from build123d import *

# Parameters (mm, degrees)
CROQUIS1_R              = 5.5
SALIENTE_EXTRUIR1_DEPTH = 4


with BuildPart() as part:
    # Croquis1 → Saliente-Extruir1 (new body)
    with BuildSketch(Plane.XY):
        Polygon((2.080750103, 8.567708442), (-6.379478111, 6.085836669), (-8.460228214, -2.481871773), (-2.080750103, -8.567708442), (6.379478111, -6.085836669), (8.460228214, 2.481871773), align=None)
        Circle(CROQUIS1_R, mode=Mode.SUBTRACT)
    extrude(amount=-SALIENTE_EXTRUIR1_DEPTH)


solid = part.part
Geometry check sheet. Reference: the model listing, model coordinates, mm. Round coordinates to 2 decimals unless told otherwise and drop trailing zeros. Order: outer loops, then holes, each group sorted by start corner. A loop starts at its lowest first (then second) coordinate and runs counter-clockwise, first axis right, second up. Notation, with made-up numbers: (62, -25.75) - (66, -25.75) arc R37 ccw to (66, 13.25) - close; hole circle Ø6 at (27, 65). An arc over 180 degrees is marked (long way). One line per question, with ' | ' between items. Start each with the question number.
(1) Depth check by flat-ended pin: pin 1 Ø1 at (x, z) = (-3.5, -3.5) entering from +Y; pin 2 Ø2 at (y, z) = (0, -0.5) entering from -X. Enter the tip coordinate at first touch or a pass-through.
(2) Sectioned sample at C-C on x = 0. Record the cut outline in (y, z).
(3) Sectioned sample at D-D on x = 6. Record the cut outline in (y, z), and give its area (3 significant figures).
(4) Sectioned sample at B-B on z = -0.85. Record the cut outline in (x, y).
(5) Sectioned sample at A-A on y = -1.25. Record the cut outline in (x, z).
(6) Thickness scan on L1, parallel to Y at x = 0, z = -1.15; L2, parallel to X at y = -4.5, z = -0.65; L3, parallel to Y at x = -2.75, z = -1.6. Record the ranges inside material, lowest first. Write a range as [from, to].
(7) Release check for a two-part mould opening along Y. For faces 1 (the cylindrical face through (-1.19, -5.37, -1.97)), 2 (the flat face through (5.32, 5.48, -1.97)), 3 (the flat face through (7.405, -1.862, -1.972)) record: released by +Y, released by -Y, zero draft, split by the parting line, or undercut.
Conclusion:
1) pin 1: stops at y = 7.08 | pin 2: stops at x = -8.1
2) outline: (-7.96, -4) - (-5.5, -4) - (-5.5, 0) - (-7.96, 0) - close; (5.5, -4) - (7.96, -4) - (7.96, 0) - (5.5, 0) - close
3) outline: (-6.2, -4) - (4.83, -4) - (4.83, 0) - (-6.2, 0) - close | area: 44.1 mm2
4) outline: (-8.46, -2.48) - (-2.08, -8.57) - (6.38, -6.09) - (8.46, 2.48) - (2.08, 8.57) - (-6.38, 6.09) - close; hole circle Ø11 at (0, 0)
5) outline: (-8.16, -4) - (-5.36, -4) - (-5.36, 0) - (-8.16, 0) - close; (5.36, -4) - (7.55, -4) - (7.55, 0) - (5.36, 0) - close
6) L1: y = [-7.96, -5.5], [5.5, 7.96] | L2: x = [-6.34, -3.16], [3.16, 6.76] | L3: y = [-7.93, -4.76], [4.76, 7.15]
7) face 1: undercut | face 2: released by +Y | face 3: released by -Y
